from build123d import *

# Parameters (mm, degrees)
SKETCH_W        = 59.5
SKETCH_H        = 22.5
PAD_DEPTH       = 1.7
SKETCH001_W     = 56.7
SKETCH001_H     = 20.7
PAD001_DEPTH    = 0.9
SKETCH002_W     = 10.5
SKETCH002_H     = 5.15
POCKET_DEPTH    = 0.7
POCKET001_DEPTH = 0.6
SKETCH004_R     = 1.65
POCKET002_DEPTH = 1.901
FILLET_R        = 2


with BuildPart() as part:
    # Sketch → Pad (new body)
    with BuildSketch(Plane.XY):
        Rectangle(SKETCH_W, SKETCH_H)
    extrude(amount=PAD_DEPTH)

    # Sketch001 (on Face6 of Pad) → Pad001 (join)
    with BuildSketch(Plane.XY.offset(1.7)):
        Rectangle(SKETCH001_W, SKETCH001_H)
    extrude(amount=PAD001_DEPTH)

    # Sketch002 (on Face4 of Pad001) → Pocket (cut)
    with BuildSketch(Plane(origin=(0, 0, 0), x_dir=(1, 0, 0), z_dir=(0, 0, -1))):
        Polygon((3.175426, 4.175), (1.587713, 6.925), (-1.587713, 6.925), (-3.175426, 4.175), (-1.587713, 1.425), (1.587713, 1.425), align=None)
        with Locations((0, -1.65)):
            Rectangle(SKETCH002_W, SKETCH002_H)
    extrude(amount=-POCKET_DEPTH, mode=Mode.SUBTRACT)

    # Sketch003 (on Face21 of Pocket) → Pocket001 (cut)
    with BuildSketch(Plane(origin=(0, 0, 0.7), x_dir=(1, 0, 0), z_dir=(0, 0, -1))):
        with BuildLine():
            ThreePointArc((-2.5, 0.85), (-5, -1.65), (-2.5, -4.15))
            Line((-2.5, -4.15), (2.5, -4.15))
            ThreePointArc((2.5, -4.15), (5, -1.65), (2.5, 0.85))
            Line((-2.5, 0.85), (2.5, 0.85))
        make_face()
    extrude(amount=-POCKET001_DEPTH, mode=Mode.SUBTRACT)

    # Sketch004 (on Face22 of Pocket001) → Pocket002 (cut, through all)
    with BuildSketch(Plane(origin=(0, 0, 0.7), x_dir=(1, 0, 0), z_dir=(0, 0, -1))):
        with Locations((0, 4.175)):
            Circle(SKETCH004_R)
        with BuildLine():
            ThreePointArc((-2.5, 0.35), (-4.5, -1.65), (-2.5, -3.65))
            Line((-2.5, -3.65), (2.5, -3.65))
            ThreePointArc((2.5, -3.65), (4.5, -1.65), (2.5, 0.35))
            Line((-2.5, 0.35), (2.5, 0.35))
        make_face()
    extrude(amount=-POCKET002_DEPTH, mode=Mode.SUBTRACT)

    # Fillet
    fillet_edges = [part.edges().sort_by_distance(p)[0] for p in [
        (-29.75, -11.25, 0.85),
        (-28.35, -10.35, 2.15),
        (-29.75, 11.25, 0.85),
        (-28.35, 10.35, 2.15),
        (28.35, -10.35, 2.15),
        (29.75, -11.25, 0.85),
        (28.35, 10.35, 2.15),
        (29.75, 11.25, 0.85),
    ]]
    fillet(fillet_edges, radius=FILLET_R)


solid = part.part
The listing builds one solid part. Answer for the finished solid, in the listing's coordinates (mm). A direction names the side the tool comes from. Round coordinates to 2 decimals unless told otherwise and drop trailing zeros. Write each loop counter-clockwise with the first axis right and the second up, starting at its lowest first coordinate (ties: lowest second). Pieces come first, ordered by that corner, then holes. Notation, with made-up numbers: (14, 69) - (30, 69) arc R17 ccw to (30, 93) - close; hole circle Ø6 at (26, -29). An arc over 180 degrees is marked (long way). Use one line per item in the form item = value. Start each with the question number.
Item 1: Find the intervals of material crossed by line 1 (Y direction, x = 0, z = 2) (3 decimals); line 2 (Y direction, x = 0, z = 1.35) (3 decimals); line 3 (X direction, y = 1.5, z = 1.5), in increasing order. Write a range as [from, to].
Item 2: A cutting plane is placed at B-B (y = 1.65). Write down the section's boundary in (x, z), plus the area to 3 significant figures.
Item 3: Flat-ended cylindrical pins translate along their axes: pin 1 Ø1.4 at (x, z) = (-0.5, 2) entering from +Y; pin 2 Ø4.5 at (x, y) = (0, -4.5) entering from -Z; pin 3 Ø0.5 at (y, z) = (-2.5, 2.5) entering from -X. Find the tip coordinate at first contact, or state that the pin passes through.
Item 4: A cutting plane is placed at D-D (y = 6.5). Write down the section's boundary in (x, z), plus the area to 3 significant figures.
Item 5: A cutting plane is placed at A-A (x = 0). Write down the section's boundary in (y, z) (3 decimals).
Item 6: Determine the mould class of faces 1 (the flat face through (-2.37, -5.57, 0.35)), 2 (the flat face through (-29.75, 0, 1)), 3 (the flat face through (0, 11.25, 1)) for opening direction X: +X half, -X half, draft (parallel to the pull), parting line (faces both ways), or undercut.
Item 7: A cutting plane is placed at C-C (x = -7.5). Write down the section's boundary in (y, z), plus the area to 3 significant figures.
Item 8: A tool of negligible diameter and unlimited length cuts with its end or side. For faces 4 (the cylindrical face through (-27.75, 9.78, 2.16)), 5 (the flat face through (-2.393, -2.819, 0.345)), 6 (the cylindrical face through (27.75, -9.78, 2.16)), 7 (the flat face through (0, -0.35, 2)), from which of +Z, -Z, +X, -X, +Y, -Y can it reach the whole face along a straight path? Write none if from no direction.
The answers:
q1.line_1 = [-10.35, -5.825], [-2.525, -0.35], [3.65, 10.35]
q1.line_2 = [-11.25, -5.825], [-2.525, -0.35], [3.65, 11.25]
q1.line_3 = [-29.75, -4.49], [4.49, 29.75]
q2.outline = (-29.75, 0) - (-5.25, 0) - (-5.25, 0.7) - (-5, 0.7) - (-5, 1.3) - (-4.5, 1.3) - (-4.5, 2.6) - (-28.35, 2.6) - (-28.35, 1.7) - (-29.75, 1.7) - close; (4.5, 1.3) - (5, 1.3) - (5, 0.7) - (5.25, 0.7) - (5.25, 0) - (29.75, 0) - (29.75, 1.7) - (28.35, 1.7) - (28.35, 2.6) - (4.5, 2.6) - close
q2.area = 127 mm^2
q3.pin_1 = 11.25
q3.pin_2 = 0.7
q3.pin_3 = -28.35
q4.outline = (-29.75, 0) - (29.75, 0) - (29.75, 1.7) - (28.35, 1.7) - (28.35, 2.6) - (-28.35, 2.6) - (-28.35, 1.7) - (-29.75, 1.7) - close
q4.area = 152 mm^2
q5.outline = (-11.25, 0) - (-6.925, 0) - (-6.925, 0.7) - (-5.825, 0.7) - (-5.825, 2.6) - (-10.35, 2.6) - (-10.35, 1.7) - (-11.25, 1.7) - close; (-2.525, 0.7) - (-1.425, 0.7) - (-1.425, 0) - (-0.925, 0) - (-0.925, 0.7) - (-0.85, 0.7) - (-0.85, 1.3) - (-0.35, 1.3) - (-0.35, 2.6) - (-2.525, 2.6) - close; (3.65, 1.3) - (4.15, 1.3) - (4.15, 0.7) - (4.225, 0.7) - (4.225, 0) - (11.25, 0) - (11.25, 1.7) - (10.35, 1.7) - (10.35, 2.6) - (3.65, 2.6) - close
q6.face_1 = undercut
q6.face_2 = -X half
q6.face_3 = draft
q7.outline = (-11.25, 0) - (11.25, 0) - (11.25, 1.7) - (10.35, 1.7) - (10.35, 2.6) - (-10.35, 2.6) - (-10.35, 1.7) - (-11.25, 1.7) - close
q7.area = 56.9 mm^2
q8.face_4 = +Z, -X, +Y
q8.face_5 = -Z
q8.face_6 = +Z, +X, -Y
q8.face_7 = +Z, -Z
